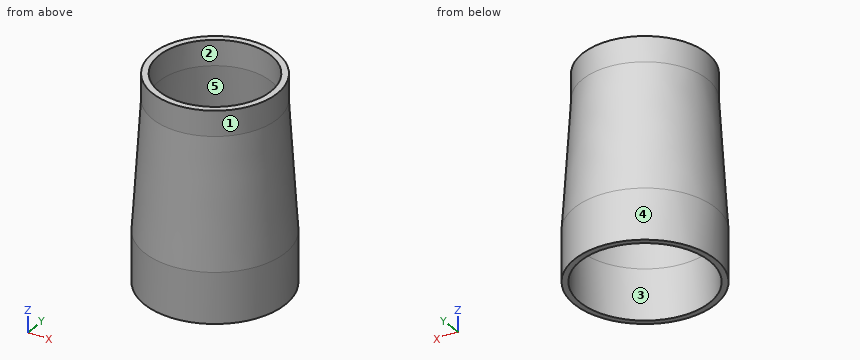
from build123d import *

# Parameters (mm, degrees)
F3_R      = 12.3698
F4_R      = 13.97
F1_R      = 11.1
F2_R      = 12.827
F7_DEPTH  = 5
F8_DEPTH  = 25.4
F9_DEPTH  = 10
F10_DEPTH = 25.4


with BuildPart() as f5:
    # F3 (on offset) → F5 section 0
    with BuildSketch(Plane.XY.offset(25.4)):
        Circle(F3_R)
    # F4 (on Top) → F5 section 1
    with BuildSketch(Plane.XY):
        Circle(F4_R)
    loft()

    # F1 (on offset) → F6 section 0
    with BuildSketch(Plane.XY.offset(25.4)):
        Circle(F1_R)
    # F2 (on Top) → F6 section 1
    with BuildSketch(Plane.XY):
        Circle(F2_R)
    loft(mode=Mode.SUBTRACT)

    # F3 (on offset) → F7 (join)
    with BuildSketch(Plane.XY.offset(25.4)):
        Circle(F3_R)
    extrude(amount=F7_DEPTH)

    # F1 (on offset) → F8 (cut)
    with BuildSketch(Plane.XY.offset(25.4)):
        Circle(F1_R)
    extrude(amount=F8_DEPTH, mode=Mode.SUBTRACT)

    # F4 (on Top) → F9 (join)
    with BuildSketch(Plane.XY):
        Circle(F4_R)
    extrude(amount=-F9_DEPTH)

    # F2 (on Top) → F10 (cut)
    with BuildSketch(Plane.XY):
        Circle(F2_R)
    extrude(amount=-F10_DEPTH, mode=Mode.SUBTRACT)


solid = f5.part
For this review, take the finished solid that the model builds, in its own axes (mm). Face numbers are marked on the shaded views. A direction names the side the tool comes from. Give positions to 0.01 mm unless a question says otherwise; leave off trailing zeros. Loops run counter-clockwise (first coordinate to the right, second up) from the corner with the lowest first, then second, coordinate; pieces in that order, holes last. Notation, with made-up numbers: M 8.5,19 L 17.5,19 A16 cw 17.5,36 Z; hole C 27,10.25 d2. An arc over 180 degrees is marked long. Put each result on its own line as item: value. Start each with the question number.
(1) For pin 1 (1 mm diameter, centred on x = -6, z = -4.5, fed in from +Y); pin 2 (12 mm diameter, centred on x = -9.5, z = 14, fed in from +Y); pin 3 (8 mm diameter, centred on y = 0.5, z = 8.5, fed in from +X), all flat-tipped, find the tip position at first contact; note any pin that passes through.
(2) The part is to be moulded in two halves that separate along X. For the marked faces 4 and 5, say which applies: +X half, -X half, draft (parallel to the pull), parting line (faces both ways), or undercut.
(3) Machinability: for the marked faces 1, 2 and 3, which of the approach directions +Z, -Z, +X, -X, +Y, -Y give a long, thin tool a straight path to every point of the face, cutting with its end or side? Answer none if there is none.
(4) Wall thickness on L1, parallel to Y at x = 0, z = -3; L2, parallel to Y at x = 0, z = 26.8; L3, parallel to X at y = 1, z = 13: over which ranges is each line inside the solid? List them lowest first.
(5) Add section C-C, the plane z = 3. Write out the cut boundary in (x, y), then the cut area to 3 significant figures.
(6) Add section B-B, the plane z = 28. Write out the cut boundary in (x, y).
(7) Add section A-A, the plane x = 0. Write out the cut boundary in (y, z), then the cut area to 3 significant figures.
Result:
1. pin 1: stops at y = 12.84
1. pin 2: stops at y = 12.66
1. pin 3: stops at x = 13.68
2. face 4: parting line
2. face 5: undercut
3. face 1: +Z
3. face 2: +Z, -Z
3. face 3: -Z
4. L1: y = -13.97 to -12.83, 12.83 to 13.97
4. L2: y = -12.37 to -11.1, 11.1 to 12.37
4. L3: x = -13.11 to -11.9, 11.9 to 13.11
5. outline: C 0,0 d27.56; hole C 0,0 d25.25
5. area: 96.1 mm^2
6. outline: C 0,0 d24.74; hole C 0,0 d22.2
7. outline: M -13.97,-10 L -12.83,-10 L -12.83,0 L -11.1,25.4 L -11.1,30.4 L -12.37,30.4 L -12.37,25.4 L -13.97,0 Z; M 11.1,25.4 L 12.83,0 L 12.83,-10 L 13.97,-10 L 13.97,0 L 12.37,25.4 L 12.37,30.4 L 11.1,30.4 Z
7. area: 96.8 mm^2
